Source: CAD feature listing. Evaluate the final solid. Frame: model axes, mm. Face numbers are marked on the shaded views. A direction names the side the tool comes from. Round coordinates to 2 decimals unless told otherwise and drop trailing zeros. Write each loop counter-clockwise with the first axis right and the second up, starting at its lowest first coordinate (ties: lowest second). Pieces come first, ordered by that corner, then holes.
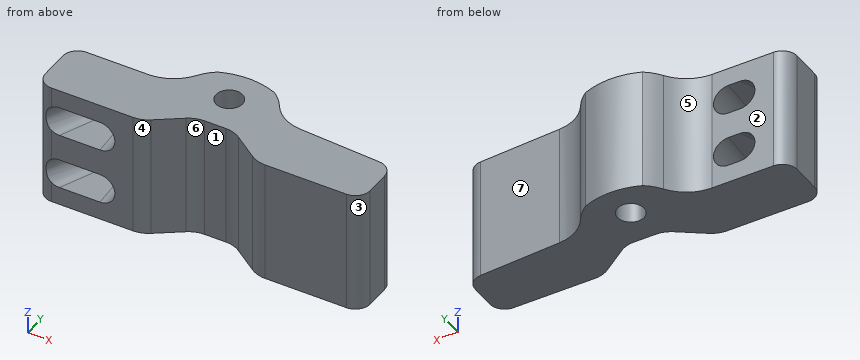
Autodesk Inventor part; units mm, degrees
ref_plane "YZ Plane" through (0, 0, 0) normal (1, 0, 0) x (0, 1, 0)
ref_plane "XZ Plane" through (0, 0, 0) normal (0, 1, 0) x (-1, 0, 0)
ref_plane "XY Plane" through (0, 0, 0) normal (0, 0, 1) x (1, 0, 0)
sketch "Sketch1" plane through (0, 0, 0) normal (0, 0, 1) x (1, 0, 0)
  line L0 (0, 0) -> (51.4289, 0) construction
  line L1 (51.4289, 0) -> (51.4289, -25.9828) construction
  line L2 (51.4289, -25.9828) -> (0, -25.9828) construction
  line L3 (0, -25.9828) -> (0, 0) construction
  circle A0 centre (24.9, -9.85) radius 2
  line L4 (1.6, -19.55) -> (1.6, -10.65)
  line L5 (1.6, -10.65) -> (13.1, -10.65)
  line L6 (1.6, -19.55) -> (17.4, -19.55)
  line L7 (17.4, -19.55) -> (23.2, -15.45)
  line L8 (23.2, -15.45) -> (29, -15.45)
  line L9 (29, -15.45) -> (34.8, -19.55)
  line L10 (34.8, -19.55) -> (50.6, -19.55)
  line L11 (50.6, -19.55) -> (50.6, -11.55)
  line L12 (50.6, -11.55) -> (36.1, -10.6377)
  arc A1 (31.1534, -7.6382) -> (29.195, -5.6092) centre (25.0705, -11.55) ccw
  arc A2 (20.6046, -5.6092) -> (18.6461, -7.6382) centre (24.7291, -11.55) ccw
  arc A3 (31.1534, -7.6382) -> (36.1, -10.6377) centre (36.4916, -4.4135) ccw
  arc A4 (13.1, -10.65) -> (18.6461, -7.6382) centre (13.1, -4.0375) ccw
  ellipse E0 centre (24.9, -20.05) end of major axis (24.9008, -35.35) minor radius 13 (29.195, -5.6092) -> (20.6046, -5.6092) ccw
  dimension "d45" = 13
  dimension "d46" = 15.3
  dimension "d22" = 4
  dimension "d35" = 0.5
  dimension "d36" = 1.6
  dimension "d37" = 10.65
  dimension "d38" = 8.9
  dimension "d39" = 3.6
  dimension "d47" = 8
  dimension "d51" = 17.4
  dimension "d52" = 25.7
  dimension "d53" = 9.7
  dimension "d54" = 11.5
  dimension "d55" = 14.5
  dimension "d57" = 0.3414
  dimension "d59" = 5.8
  dimension "d61" = 4.1
  dimension "d63" = 15.8
  dimension "d64" = 15.8
  dimension "d66" = 8
  dimension "d72" = 0.1705
  dimension "d76" = 7.2322
  dimension "d77" = 6.2366
extrude "Extrusion1" add sketch "Sketch1" along normal blind 18.5
fillet "Fillet1" radius 2.25 4 edges at (1.6, -10.65, 9.25) (1.6, -19.55, 9.25) (50.6, -11.55, 9.25) (50.6, -19.55, 9.25)
fillet "Fillet2" radius 4 4 edges at (23.2, -15.45, 9.25) (29, -15.45, 9.25) (34.8, -19.55, 9.25) (17.4, -19.55, 9.25)
sketch "Sketch3" plane through (3.85, -19.55, 0) normal (0, -1, 0) x (1, 0, 0)
  line L0 (0, 18.5) -> (12.279, 18.5)
  line L1 (12.279, 0) -> (0, 0)
  line L2 (1.21, 13.5) -> (7.31, 13.5) construction
  line L3 (1.21, 11.25) -> (7.31, 11.25)
  line L4 (7.31, 15.75) -> (1.21, 15.75)
  arc A0 (1.21, 15.75) -> (1.21, 11.25) centre (1.21, 13.5) ccw
  arc A1 (7.31, 11.25) -> (7.31, 15.75) centre (7.31, 13.5) ccw
  line L5 (1.21, 5) -> (7.31, 5) construction
  line L6 (1.21, 7.25) -> (7.31, 7.25)
  line L7 (7.31, 2.75) -> (1.21, 2.75)
  arc A2 (1.21, 7.25) -> (1.21, 2.75) centre (1.21, 5) ccw
  arc A3 (7.31, 2.75) -> (7.31, 7.25) centre (7.31, 5) ccw
  line L8 (-2.25, 18.5) -> (-2.25, 0)
  point P0 (-3.85, 0)
  point P1 (4.26, 13.5)
  point P2 (4.26, 5)
  dimension "d88" = 4.5
  dimension "d89" = 6.1
  dimension "d90" = 5
  dimension "d91" = 5
  dimension "d92" = 9.56
sketch "Sketch2" plane through (13.1, -10.65, 18.5) normal (0, 1, 0) x (1, 0, 0)
  line L0 (0, 0) -> (-9.25, 0)
  line L1 (-9.25, 18.5) -> (0, 18.5)
  line L2 (-4.205, 13.5) -> (-2.455, 13.5) construction
  line L3 (-4.205, 11.25) -> (-2.455, 11.25)
  line L4 (-2.455, 15.75) -> (-4.205, 15.75)
  arc A0 (-4.205, 15.75) -> (-4.205, 11.25) centre (-4.205, 13.5) ccw
  arc A1 (-2.455, 11.25) -> (-2.455, 15.75) centre (-2.455, 13.5) ccw
  line L5 (-4.205, 5) -> (-2.455, 5) construction
  line L6 (-4.205, 2.75) -> (-2.455, 2.75)
  line L7 (-2.455, 7.25) -> (-4.205, 7.25)
  arc A2 (-4.205, 7.25) -> (-4.205, 2.75) centre (-4.205, 5) ccw
  arc A3 (-2.455, 2.75) -> (-2.455, 7.25) centre (-2.455, 5) ccw
  line L8 (-11.5, 18.5) -> (-11.5, 0)
  point P0 (-13.1, 18.5)
  point P1 (-3.33, 13.5)
  point P2 (-3.33, 5)
  dimension "d83" = 4.5
  dimension "d84" = 1.75
  dimension "d85" = 5
  dimension "d86" = 5
  dimension "d87" = 8.17
loft "Loft1" cut profiles "Sketch3", "Sketch2" contours A0 L4 A1 L3 / A2 L7 A3 L6
loft "Loft2" cut profiles "Sketch3", "Sketch2" contours L6 A3 L7 A2 / A0 L4 A1 L3
properties part number "FelixOriginalLever"
Q1. Section query B-B, the plane z = 13.75. Give the number of separate pieces and of enclosed holes in the cut face, and give its area (3 significant figures).
Q2. Set-up query: the marked faces 1, 2 and 3. Return all of +Z, -Z, +X, -X, +Y, -Y with unobstructed straight access to the full face (end or side cutting, diameter ignored); none if empty.
Q3. Section query D-D, the plane x = 33. Output: boundary loops of the cut face in (y, z).
Q4. Mould query, pull axis X, two halves, no side actions, for the marked faces 4, 5, 6 and 7. Classes: pulls with the +X half, pulls with the -X half, needs draft (parallel to the pull), parting line crosses it, or undercut.
Q5. Pin query (flat end, axial travel): P1, Ø1.6, axis at x = 26, z = 7, coming from the -Y side; P2, Ø3, axis at x = 33.5, z = 9.5, coming from the +Y side; P3, Ø5, axis at y = -6.5, z = 12, coming from the +X side. Return the tip coordinate at first contact, or that it passes through.
Q6. Line query: line 1 (Y direction, x = 24.9, z = 5.25); line 2 (X direction, y = -16.5, z = 9.25); line 3 (X direction, y = -18.5, z = 9.25). Output: solid intervals per line, ascending.
Q7. Section query A-A, the plane y = -9.85. Output: boundary loops of the cut face in (x, z).
Filled in:
1. separate pieces: 2
1. enclosed holes: 1
1. area: 365 mm2
2. face 1: +Z, -Z, -Y
2. face 2: +Z, -Z, -X, +Y
2. face 3: +Z, -Z, +X, -Y
3. outline: (-18.28, 0) - (-9.58, 0) - (-9.58, 18.5) - (-18.28, 18.5) - close
4. face 4: undercut
4. face 5: pulls with the -X half
4. face 6: undercut
4. face 7: pulls with the +X half
5. P1: stops at y = -15.45
5. P2: stops at y = -8.74
5. P3: stops at x = 32.27
6. line 1: y = -15.45 to -11.85, -7.85 to -4.75
6. line 2: x = 1.6 to 21.71, 30.49 to 50.6
6. line 3: x = 1.95 to 18.89, 33.31 to 50.25
7. outline: (16.25, 0) - (22.9, 0) - (22.9, 18.5) - (16.25, 18.5) - close; (26.9, 0) - (33.44, 0) - (33.44, 18.5) - (26.9, 18.5) - close
